from build123d import *

# Parameters (mm, degrees)
SCHIZZO1_W                   = 20.5
SCHIZZO1_H                   = 14.5
ESTRUSIONE_ESTRUSIONE1_DEPTH = 1.75
SCHIZZO2_W                   = 17
SCHIZZO2_H                   = 12
ESTRUSIONE_ESTRUSIONE2_DEPTH = 10.75
SCHIZZO3_W                   = 3
SCHIZZO3_H                   = 12
ESTRUSIONE_ESTRUSIONE3_DEPTH = 1
SCHIZZO4_W                   = 3
SCHIZZO4_H                   = 12
ESTRUSIONE_ESTRUSIONE4_DEPTH = 1
SCHIZZO6_W                   = 8.25
SCHIZZO6_H                   = 10.5
ESTRUSIONE_ESTRUSIONE5_DEPTH = 0.5
ESTRUSIONE_ESTRUSIONE6_DEPTH = 10.5
SCHIZZO9_W                   = 0.5
SCHIZZO9_H                   = 4
ESTRUSIONE_ESTRUSIONE7_DEPTH = 8


with BuildPart() as part:
    # Schizzo1 → Estrusione-Estrusione1 (new body)
    with BuildSketch(Plane.XY):
        Rectangle(SCHIZZO1_W, SCHIZZO1_H)
    extrude(amount=ESTRUSIONE_ESTRUSIONE1_DEPTH)

    # Schizzo2 → Estrusione-Estrusione2 (add)
    with BuildSketch(Plane(origin=(0, 0, 0), x_dir=(-1, 0, 0), z_dir=(0, 0, -1))):
        Rectangle(SCHIZZO2_W, SCHIZZO2_H)
    extrude(amount=ESTRUSIONE_ESTRUSIONE2_DEPTH)

    # Schizzo3 → Estrusione-Estrusione3 (add)
    with BuildSketch(Plane(origin=(8.5, 0, 0), x_dir=(0, 0, -1), z_dir=(1, 0, 0))):
        with Locations((10.25, 0)):
            Rectangle(SCHIZZO3_W, SCHIZZO3_H)
    extrude(amount=ESTRUSIONE_ESTRUSIONE3_DEPTH)

    # Schizzo4 → Estrusione-Estrusione4 (add)
    with BuildSketch(Plane.ZY.offset(8.5)):
        with Locations((-10.25, 0)):
            Rectangle(SCHIZZO4_W, SCHIZZO4_H)
    extrude(amount=ESTRUSIONE_ESTRUSIONE4_DEPTH)

    # Schizzo6 → Estrusione-Estrusione5 (add)
    with BuildSketch(Plane.XY.offset(1.75)):
        with Locations((-4.125, 0)):
            Rectangle(SCHIZZO6_W, SCHIZZO6_H)
    extrude(amount=ESTRUSIONE_ESTRUSIONE5_DEPTH)

    # Schizzo8 → Estrusione-Estrusione6 (add)
    with BuildSketch(Plane(origin=(0, 5.25, 0), x_dir=(1, 0, 0), z_dir=(0, 1, 0))):
        Polygon((0, -2.25), (6.048387887, -5.65769108), (8.25, -1.75), (0, -1.75), align=None)
    extrude(amount=-ESTRUSIONE_ESTRUSIONE6_DEPTH)

    # Schizzo9 → Estrusione-Estrusione7 (add)
    with BuildSketch(Plane(origin=(0, 0, -10.75), x_dir=(-1, 0, 0), z_dir=(0, 0, -1))):
        with Locations((7.25, 0)):
            Rectangle(SCHIZZO9_W, SCHIZZO9_H)
        with Locations((0.25, 0)):
            Rectangle(SCHIZZO9_W, SCHIZZO9_H)
    extrude(amount=ESTRUSIONE_ESTRUSIONE7_DEPTH)


solid = part.part
Here's how the part is built. I have some questions about the finished solid (model axes, mm). A direction names the side the tool comes from. Round coordinates to 2 decimals unless told otherwise and drop trailing zeros. Loops run counter-clockwise (first coordinate to the right, second up) from the corner with the lowest first, then second, coordinate; pieces in that order, holes last. Notation, with made-up numbers: (51.5, 11.5) - (103.5, 11.5) arc R29 cw to (103.5, 42.5) - close; hole circle Ø1 at (-24, 7.5). An arc over 180 degrees is marked (long way). One line per question, with ' | ' between items. Start each with the question number.
Q1. I want a section at C-C (x = -4.75). Write out the boundary of the cut face in (y, z).
Q2. I want a section at D-D (z = -7). Write out the boundary of the cut face in (x, y).
Q3. We'd pull the mould along Z, two halves only. Please class faces 1 (the flat face through (2.98, 0.07, 3.93)), 2 (the flat face through (2, 5.25, 3)), 3 (the flat face through (-8.5, 0, -4)): +Z half, -Z half, draft (parallel to the pull), parting line (faces both ways), or undercut.
Q4. Please list where these lines run through material, in increasing order: line 1 (Y direction, x = -5, z = -3.5); line 2 (X direction, y = 1.5, z = -8.5); line 3 (Z direction, x = -0.75, y = 5.75). Write a range as [from, to].
Q5. I want a section at B-B (z = -12.75). Write out the boundary of the cut face in (x, y), then the cut area to 3 significant figures.
Q6. Will these pins go through, and if not, where does the flat tip stop? pin 1 (4.5 mm diameter, centred on x = 1, y = 2.5, fed in from -Z); pin 2 (0.9 mm diameter, centred on y = 3, z = -11, fed in from -X); pin 3 (6.5 mm diameter, centred on x = -5, y = 0.5, fed in from +Z); pin 4 (1 mm diameter, centred on x = 1, y = 5.5, fed in from -Z).
Q7. For faces 4 (the flat face through (-0.1, -6.3, 0)), 5 (the flat face through (0, 6, -6)), 6 (the flat face through (-9, 0, -8.75)), 7 (the flat face through (-7, 0, -15)), which set-ups out of +Z, -Z, +X, -X, +Y, -Y let a thin tool reach every point of the face, with its end or its side?
Response values:
1) outline: (-7.25, 0) - (-6, 0) - (-6, -10.75) - (6, -10.75) - (6, 0) - (7.25, 0) - (7.25, 1.75) - (5.25, 1.75) - (5.25, 2.25) - (-5.25, 2.25) - (-5.25, 1.75) - (-7.25, 1.75) - close
2) outline: (-8.5, -6) - (8.5, -6) - (8.5, 6) - (-8.5, 6) - close
3) face 1: +Z half | face 2: draft | face 3: undercut
4) line 1: y = [-6, 6] | line 2: x = [-8.5, 8.5] | line 3: z = [-10.75, 1.75]
5) outline: (-7.5, -2) - (-7, -2) - (-7, 2) - (-7.5, 2) - close; (-0.5, -2) - (0, -2) - (0, 2) - (-0.5, 2) - close | area: 4.00 mm²
6) pin 1: stops at z = -18.75 | pin 2: stops at x = -9.5 | pin 3: stops at z = 2.25 | pin 4: stops at z = -10.75
7) face 4: none | face 5: -Z, +X, -X, +Y | face 6: -X, +Y, -Y | face 7: -Z, +Y, -Y
